Check sheet for the drawn part. Datum: minimum x, y, z corner. Units: mm. Coordinates: 2 decimals unless noted, no trailing zeros. Write each loop counter-clockwise with the first axis right and the second up, starting at its lowest first coordinate (ties: lowest second). Pieces come first, ordered by that corner, then holes. Notation, with made-up numbers: M -37,14 L -25,14 A23 cw -25,41 Z; hole C 20,48.5 d5. An arc over 180 degrees is marked long. Write item = value, one per line. Start each with the question number.
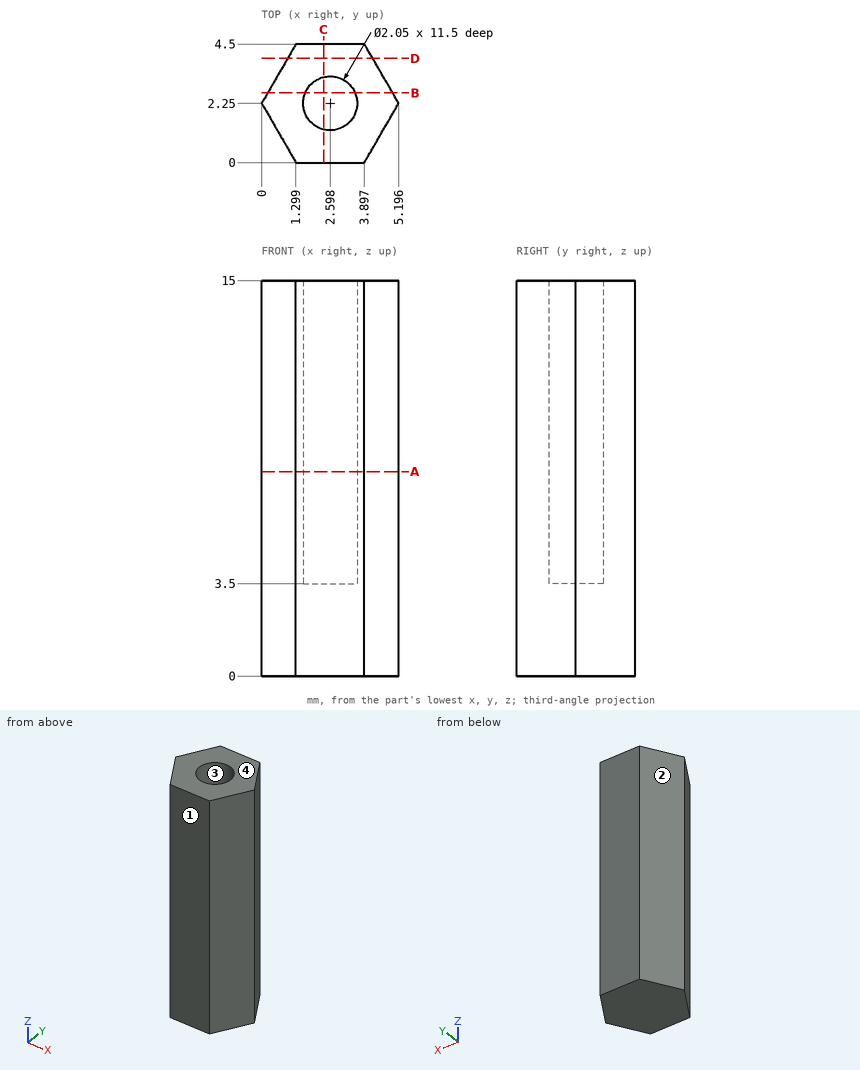
Q1. Draft check along Y on the marked faces 1, 2, 3 and 4. Enter one of: pulls with the +Y half, pulls with the -Y half, needs draft (parallel to the pull), parting line crosses it, or undercut.
Q2. Cross-section at A-A on z = 7.75. Enter the section's corners in (x, y) (3 decimals), and give its area (3 significant figures).
Q3. Cross-section at D-D on y = 3.95. Enter the section's corners in (x, z), and give its area (3 significant figures).
Q4. Cross-section at B-B on y = 2.65. Enter the section's corners in (x, z) (1 decimal), and give its area (3 significant figures).
Q5. Scan lines: L1, parallel to Y at x = 2.55, z = 4.5; L2, parallel to Y at x = 2.35, z = 11 (1 decimal); L3, parallel to X at y = 2.65, z = 13.5 (1 decimal). Record each from-to range of solid material in increasing order.
Q6. Cross-section at C-C on x = 2.35. Enter the section's corners in (y, z).
Q7. Gauge pin test, flat ends, axial feed: pin 1 (1 mm diameter, centred on x = 1.5, y = 3.5, fed in from -Z); pin 2 (0.6 mm diameter, centred on x = 2, y = 2, fed in from +Z). Record the tip position at first contact, or that the pin passes through.
Values found:
q1.face_1 = pulls with the -Y half
q1.face_2 = pulls with the +Y half
q1.face_3 = undercut
q1.face_4 = needs draft
q2.outline = M 0,2.25 L 1.299,0 L 3.897,0 L 5.196,2.25 L 3.897,4.5 L 1.299,4.5 Z; hole C 2.598,2.25 d2.05
q2.area = 14.2 mm²
q3.outline = M 0.98,0 L 4.21,0 L 4.21,15 L 0.98,15 Z
q3.area = 48.5 mm²
q4.outline = M 0.2,0 L 5,0 L 5,15 L 3.5,15 L 3.5,3.5 L 1.7,3.5 L 1.7,15 L 0.2,15 Z
q4.area = 49.3 mm²
q5.L1 = 0 to 1.23, 3.27 to 4.5
q5.L2 = 0 to 1.3, 3.2 to 4.5
q5.L3 = 0.2 to 1.7, 3.5 to 5
q6.outline = M 0,0 L 4.5,0 L 4.5,15 L 3.24,15 L 3.24,3.5 L 1.26,3.5 L 1.26,15 L 0,15 Z
q7.pin_1 = 0
q7.pin_2 = 3.5
